from build123d import *

# Parameters (mm, degrees)
SKETCH1_R           = 0.65
SKETCH1_R_2         = 3.35
SKETCH1_R_3         = 1.25
BOSS_EXTRUDE1_DEPTH = 1.4


with BuildPart() as part:
    # Sketch1 → Boss-Extrude1 (new body)
    # profile 1 of 4: a face of its own
    with BuildSketch(Plane(origin=(0, 0, 0), x_dir=(1, 0, 0), z_dir=(0, 1, 0))):
        with BuildLine():
            Line((-0.340877193, 3.332612), (-14.443333333, 1.890138149))
            ThreePointArc((-14.443333333, 1.890138149), (-12.976684119, 1.410200931), (-12.35, 0))
            ThreePointArc((-12.35, 0), (-12.976684119, -1.410200931), (-14.443333333, -1.890138149))
            Line((-14.443333333, -1.890138149), (-0.340877193, -3.332612))
            ThreePointArc((-0.340877193, -3.332612), (-3.35, 0), (-0.340877193, 3.332612))
        make_face()
    # profile 2 of 4: a face of its own
    with BuildSketch(Plane(origin=(0, 0, 0), x_dir=(1, 0, 0), z_dir=(0, 1, 0))):
        with BuildLine():
            ThreePointArc((-12.35, 0), (-12.976684119, 1.410200931), (-14.443333333, 1.890138149))
            ThreePointArc((-14.443333333, 1.890138149), (-16.15, 0), (-14.443333333, -1.890138149))
            ThreePointArc((-14.443333333, -1.890138149), (-12.976684119, -1.410200931), (-12.35, 0))
        make_face()
        with Locations(Location((-14.5, 0, 0), (0, 0, 270))):
            Circle(SKETCH1_R, mode=Mode.SUBTRACT)
    # profile 3 of 4: a face of its own
    with BuildSketch(Plane(origin=(0, 0, 0), x_dir=(1, 0, 0), z_dir=(0, 1, 0))):
        Circle(SKETCH1_R_2)
        with Locations(Location((0, 0, 0), (0, 0, 270))):
            Circle(SKETCH1_R_3, mode=Mode.SUBTRACT)
    # profile 4 of 4: a face of its own
    with BuildSketch(Plane(origin=(0, 0, 0), x_dir=(1, 0, 0), z_dir=(0, 1, 0))):
        with BuildLine():
            ThreePointArc((3.35, 0), (2.245056948, 2.486406905), (-0.340877193, 3.332612))
            ThreePointArc((-0.340877193, 3.332612), (-3.35, 0), (-0.340877193, -3.332612))
            ThreePointArc((-0.340877193, -3.332612), (2.245056948, -2.486406905), (3.35, 0))
        make_face()
        with Locations(Location((0, 0, 0), (0, 0, 270))):
            Circle(SKETCH1_R_3, mode=Mode.SUBTRACT)
    extrude(amount=BOSS_EXTRUDE1_DEPTH)


solid = part.part
CAD build for the part. Positions are in the model's coordinates, mm. Coordinates: 2 decimals unless noted, no trailing zeros. Write each loop counter-clockwise with the first axis right and the second up, starting at its lowest first coordinate (ties: lowest second). Pieces come first, ordered by that corner, then holes. Notation, with made-up numbers: M 23,-15 L 82,-15 A18 cw 82,12 Z; hole C -34.75,67.5 d7. An arc over 180 degrees is marked long. Return JSON: item names as keys, results as strings.
Item 1: Slice it at A-A, the plane x = 0. Write the cut outline in (y, z), and give its area (3 significant figures).
Findings below:
{"outline": "M 0,-3.35 L 1.4,-3.35 L 1.4,-1.25 L 0,-1.25 Z; M 0,1.25 L 1.4,1.25 L 1.4,3.35 L 0,3.35 Z", "area": "5.88 mm2"}
Item 2: Drop flat-ended pins along their axis: pin 1 Ø3 at (x, z) = (0, 0) entering from +Y; pin 2 Ø0.8 at (x, z) = (-14.5, 0) entering from +Y. Give the stop position or say it passes through.
Findings below:
{"pin 1": "stops at y = 1.4", "pin 2": "passes through"}
Item 3: Slice it at B-B, the plane y = 1.1. Write the cut outline in (x, z), and give its area (3 significant figures).
Findings below:
{"outline": "M -14.44,-1.89 L -0.34,-3.33 A3.35 ccw long -0.34,3.33 L -14.44,1.89 A1.9 ccw Z; hole C -14.5,0 d1.3; hole C 0,0 d2.5", "area": "92.3 mm2"}
Item 4: Slice it at D-D, the plane x = -12.5. Write the cut outline in (y, z), and give its area (3 significant figures).
Findings below:
{"outline": "M 0,-2.09 L 1.4,-2.09 L 1.4,2.09 L 0,2.09 Z", "area": "5.85 mm2"}
Item 5: Two-plate mould, pull along Z, no slides. Class faces 1 (the cylindrical face through (-1.22, 0.69, -0.27)), 2 (the flat face through (-7.29, 0.69, -2.62)), 3 (the cylindrical face through (-16.15, 0.69, -0.04)), 4 (the flat face through (-7.5, 0.7, 2.6)): +Z half, -Z half, draft (parallel to the pull), parting line (faces both ways), or undercut.
Findings below:
{"face 1": "undercut", "face 2": "-Z half", "face 3": "parting line", "face 4": "+Z half"}
Item 6: Slice it at C-C, the plane x = -6.5. Write the cut outline in (y, z).
Findings below:
{"outline": "M 0,-2.7 L 1.4,-2.7 L 1.4,2.7 L 0,2.7 Z"}
Item 7: Probe line 1 (X direction, y = 1.15, z = -0.5); line 2 (X direction, y = 1.1, z = -1); line 3 (Z direction, x = -10, y = 0.3). List the from-to ranges inside material, lowest first. Write a range as from..to.
Findings below:
{"line 1": "x = -16.08..-14.92, -14.08..-1.15, 1.15..3.31", "line 2": "x = -15.87..-0.75, 0.75..3.2", "line 3": "z = -2.34..2.34"}
